The model under review builds one solid part; all positions refer to its coordinate system, in mm. Give positions to 0.01 mm unless a question says otherwise; leave off trailing zeros. Loops run counter-clockwise (first coordinate to the right, second up) from the corner with the lowest first, then second, coordinate; pieces in that order, holes last. Notation, with made-up numbers: M 27,-8 L 48,-8 A19 ccw 48,-1 Z; hole C 9.25,29 d1. An arc over 180 degrees is marked long. One line per item, written item: value. Start each with the question number.
Q1. We need section A-A on z = 0. Write out the cut boundary in (x, y) (3 decimals).
Q2. To check wall thickness, follow line 1 along X through (y, z) = (-84, 0); line 2 along Z through (x, y) = (-152.5, 219). State the ranges of each line that lie inside material, in increasing order. Write a range as from..to.
Q3. Mouldability with a two-part tool opening along X and no side actions: class faces 1 (the face through (-68.974, 254.507, -219.025)), 2 (the face through (223, 255.029, 57)), 3 (the face through (226.254, 2.468, -117.68)) as released by +X, released by -X, zero draft, split by the parting line, or undercut.
Q4. We need section B-B on x = 0. Write out the cut boundary in (y, z) (3 decimals), plus the area to 3 significant figures.
Q5. For pin 1 (12 mm diameter, centred on x = -86, y = -86, fed in from +Z); pin 2 (12 mm diameter, centred on x = 69.5, y = -72, fed in from +Z); pin 3 (2 mm diameter, centred on x = -184.5, y = 17, fed in from +Z), all flat-tipped, find the tip position at first contact; note any pin that passes through.
Q6. We need section C-C on y = 80.5. Write out the cut boundary in (x, z), plus the area to 3 significant figures.
```python
from build123d import *


with BuildPart() as part:
    # Sketch8 → Revolve1 (revolve)
    with BuildSketch(Plane(origin=(0, 0, 0), x_dir=(0, 0, -1), z_dir=(1, 0, 0))):
        with BuildLine():
            Line((254, 0), (254, -254))
            Line((254, -254), (255.0287, -254))
            Line((255.0287, -254), (255.0287, 251.8537))
            ThreePointArc((255.0287, 251.8537), (254.09876403, 254.09876403), (251.8537, 255.0287))
            Line((251.8537, 255.0287), (229.6287, 255.0287))
            Line((229.6287, 255.0287), (229.6287, 254))
            Line((229.6287, 254), (250.825, 254))
            ThreePointArc((250.825, 254), (253.07006403, 253.07006403), (254, 250.825))
            Line((254, 250.825), (254, 0))
        make_face()
    revolve(axis=Axis((0, 0, 0), (0, 1, 0)))


solid = part.part
```
Solved:
1. outline: M -255.029,-254 L -254,-254 L -254,250.825 A3.175 cw -250.825,254 L -229.629,254 L -229.629,255.029 L -251.854,255.029 A3.175 ccw -255.029,251.854 Z; M 229.629,254 L 250.825,254 A3.175 cw 254,250.825 L 254,-254 L 255.029,-254 L 255.029,251.854 A3.175 ccw 251.854,255.029 L 229.629,255.029 Z
2. line 1: -255.03..-254, 254..255.03
2. line 2: -204.41..-203.12, 203.12..204.41
3. face 1: undercut
3. face 2: zero draft
3. face 3: split by the parting line
4. outline: M -254,-255.029 L 251.854,-255.029 A3.175 ccw 255.029,-251.854 L 255.029,-229.629 L 254,-229.629 L 254,-250.825 A3.175 cw 250.825,-254 L -254,-254 Z; M -254,254 L 250.825,254 A3.175 cw 254,250.825 L 254,229.629 L 255.029,229.629 L 255.029,251.854 A3.175 ccw 251.854,255.029 L -254,255.029 Z
4. area: 1,100 mm2
5. pin 1: z = 242.16
5. pin 2: z = 247
5. pin 3: z = 177.11
6. outline: C 0,0 d510.06; hole C 0,0 d508
6. area: 1,650 mm2
